Could you check a few things on this model? Use its own coordinates, in mm. A direction names the side the tool comes from. Round coordinates to 2 decimals unless told otherwise and drop trailing zeros. Loops run counter-clockwise (first coordinate to the right, second up) from the corner with the lowest first, then second, coordinate; pieces in that order, holes last.
from build123d import *

# Parameters (mm, degrees)
SKETCH_1_R          = 11.25
EXTRUDE_1_DEPTH     = 4
CHAMFER_1_SIZE      = 3
SKETCH_2_W          = 6
SKETCH_2_H          = 3
CUT_EXTRUDE_1_DEPTH = 2
EXTRUDE_2_DEPTH     = 25
SKETCH_4_R          = 6.25
EXTRUDE_3_DEPTH     = 5


with BuildPart() as part:
    # 草图1 → 拉伸1 (new body)
    with BuildSketch(Plane.XY):
        Circle(SKETCH_1_R)
    extrude(amount=EXTRUDE_1_DEPTH)

    # 倒角1
    chamfer_1_edges = [part.edges().sort_by_distance(p)[0] for p in [
        (-11.25, 0, 4),
    ]]
    chamfer(chamfer_1_edges, length=CHAMFER_1_SIZE)

    # 草图2 → 切除-拉伸1 (cut)
    with BuildSketch(Plane.XY.offset(4)):
        Rectangle(SKETCH_2_W, SKETCH_2_H)
    extrude(amount=-CUT_EXTRUDE_1_DEPTH, mode=Mode.SUBTRACT)

    # 草图3 → 拉伸2 (add)
    with BuildSketch(Plane(origin=(0, 0, 0), x_dir=(-1, 0, 0), z_dir=(0, 0, -1))):
        with BuildLine():
            Line((-7.5, 2.783882181), (-7.5, -2.783882181))
            ThreePointArc((-7.5, -2.783882181), (0, -8), (7.5, -2.783882181))
            Line((7.5, -2.783882181), (7.5, 2.783882181))
            ThreePointArc((7.5, 2.783882181), (0, 8), (-7.5, 2.783882181))
        make_face()
    extrude(amount=EXTRUDE_2_DEPTH)

    # 草图4 → 拉伸3 (add)
    with BuildSketch(Plane(origin=(0, 0, -25), x_dir=(-1, 0, 0), z_dir=(0, 0, -1))):
        Circle(SKETCH_4_R)
    extrude(amount=EXTRUDE_3_DEPTH)


solid = part.part
Item 1: Will these pins go through, and if not, where does the flat tip stop? pin 1 (2 mm diameter, centred on x = 1, z = 3.5, fed in from -Y); pin 2 (12 mm diameter, centred on x = -2.5, z = -26, fed in from -Y); pin 3 (1.6 mm diameter, centred on x = -1, z = 3, fed in from +Y).
Results list:
pin 1: stops at y = -9.7
pin 2: stops at y = -8
pin 3: stops at y = 10
Item 2: For faces 1 (the flat face through (3, 0, 3)), 2 (the cylindrical face through (0, -8, -12)), 3 (the flat face through (-7.5, 0, -12)), 4 (the flat face through (6, 3, -25)), 5 (the cylindrical face through (0, 8, -12)), which set-ups out of +Z, -Z, +X, -X, +Y, -Y let a thin tool reach every point of the face, with its end or its side?
Results list:
face 1: +Z
face 2: -Z, -Y
face 3: -Z, -X, +Y, -Y
face 4: -Z
face 5: -Z, +Y
Item 3: If we section it at C-C, the plane z = -25.5: Please give me the cut outline in (x, y), then the cut area to 3 significant figures.
Results list:
outline: circle Ø12.5 at (0, 0)
area: 123 mm2
Item 4: If we section it at B-B, the plane x = 0: Please give me the cut outline in (y, z).
Results list:
outline: (-11.25, 0) - (-8, 0) - (-8, -25) - (-6.25, -25) - (-6.25, -30) - (6.25, -30) - (6.25, -25) - (8, -25) - (8, 0) - (11.25, 0) - (11.25, 1) - (8.25, 4) - (1.5, 4) - (1.5, 2) - (-1.5, 2) - (-1.5, 4) - (-8.25, 4) - (-11.25, 1) - close
Item 5: If I drill on line 1 along X through (y, z) = (-2.5, -23.5); line 2 along Z through (x, y) = (-6.25, -4.75); line 3 along Z through (x, y) = (10.5, 2.25), over which ranges is the centre line in solid material (lowest first)?
Results list:
line 1: x = -7.5 to 7.5
line 2: z = -25 to 4
line 3: z = 0 to 1.51
Item 6: We'd pull the mould along Y, two halves only. Please class faces 6 (the flat face through (-8, 0, 0)), 7 (the flat face through (0, -1.5, 3)), 8 (the conical face through (-1.82, -8.2, 3.85)): released by +Y, released by -Y, zero draft, split by the parting line, or undercut.
Results list:
face 6: zero draft
face 7: undercut
face 8: split by the parting line
Item 7: If we section it at D-D, the plane z = -13.5: Please give me the cut outline in (x, y).
Results list:
outline: (-7.5, -2.78) arc R8 ccw to (7.5, -2.78) - (7.5, 2.78) arc R8 ccw to (-7.5, 2.78) - close
Item 8: If we section it at A-A, the plane y = 0: Please give me the cut outline in (x, z).
Results list:
outline: (-11.25, 0) - (-7.5, 0) - (-7.5, -25) - (-6.25, -25) - (-6.25, -30) - (6.25, -30) - (6.25, -25) - (7.5, -25) - (7.5, 0) - (11.25, 0) - (11.25, 1) - (8.25, 4) - (3, 4) - (3, 2) - (-3, 2) - (-3, 4) - (-8.25, 4) - (-11.25, 1) - close
